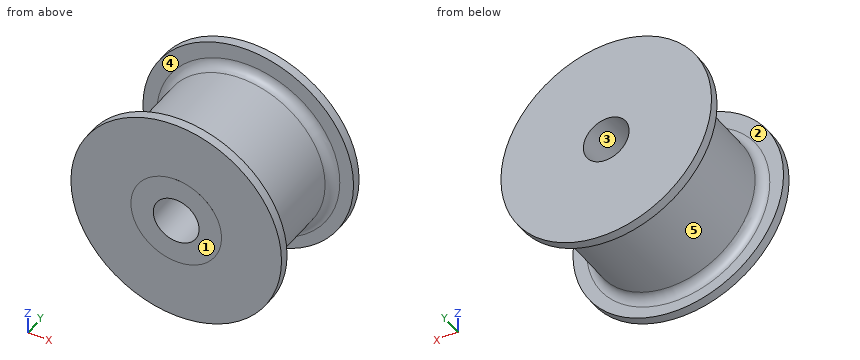
```python
from build123d import *

# Parameters (mm, degrees)
SKETCH1_R           = 4.95
BOSS_EXTRUDE2_DEPTH = 0.001
SKETCH4_R           = 11.5
BOSS_EXTRUDE3_DEPTH = 1
SKETCH5_R           = 9
BOSS_EXTRUDE4_DEPTH = 12
SKETCH6_R           = 11.5
BOSS_EXTRUDE5_DEPTH = 1
FILLET1_R           = 1
FILLET2_R           = 1
SKETCH7_R           = 2.5
CUT_EXTRUDE1_DEPTH  = 15.001


with BuildPart() as part:
    # Sketch1 → Boss-Extrude2 (new body)
    with BuildSketch(Plane(origin=(0, 0, 0), x_dir=(1, 0, 0), z_dir=(0, 1, 0))):
        Circle(SKETCH1_R)
    extrude(amount=BOSS_EXTRUDE2_DEPTH)

    # Sketch4 → Boss-Extrude3 (add)
    with BuildSketch(Plane(origin=(0, 0.001, 0), x_dir=(1, 0, 0), z_dir=(0, 1, 0))):
        Circle(SKETCH4_R)
    extrude(amount=BOSS_EXTRUDE3_DEPTH)

    # Sketch5 → Boss-Extrude4 (add)
    with BuildSketch(Plane(origin=(0, 1.001, 0), x_dir=(1, 0, 0), z_dir=(0, 1, 0))):
        with Locations((0, 0.291114712)):
            Circle(SKETCH5_R)
    extrude(amount=BOSS_EXTRUDE4_DEPTH)

    # Sketch6 → Boss-Extrude5 (add)
    with BuildSketch(Plane(origin=(0, 13.001, 0), x_dir=(1, 0, 0), z_dir=(0, 1, 0))):
        Circle(SKETCH6_R)
    extrude(amount=BOSS_EXTRUDE5_DEPTH)

    # Fillet1
    fillet1_edges = [part.edges().sort_by_distance(p)[0] for p in [
        (-9, 1.001, -0.291114712),
    ]]
    fillet(fillet1_edges, radius=FILLET1_R)

    # Fillet2
    fillet2_edges = [part.edges().sort_by_distance(p)[0] for p in [
        (-9, 13.001, -0.291114712),
    ]]
    fillet(fillet2_edges, radius=FILLET2_R)

    # Sketch7 → Cut-Extrude1 (cut, through all)
    with BuildSketch(Plane.XZ):
        Circle(SKETCH7_R)
    extrude(amount=-CUT_EXTRUDE1_DEPTH, mode=Mode.SUBTRACT)


solid = part.part
```
Here's how the part is built. I have some questions about the finished solid (model axes, mm). Face numbers are marked on the shaded views. A direction names the side the tool comes from. Give positions to 0.01 mm unless a question says otherwise; leave off trailing zeros. Loops run counter-clockwise (first coordinate to the right, second up) from the corner with the lowest first, then second, coordinate; pieces in that order, holes last. Notation, with made-up numbers: (16.5, 65) -> (57.5, 65) arc R6 cw to (57.5, 71) -> close; hole circle Ø7 at (-23.75, 42.25). An arc over 180 degrees is marked (long way). Use one line per item in the form item = value. Start each with the question number.
1) Thinking about a two-plate mould opening in Z: for the marked faces 3, 4 and 5, which applies, +Z half, -Z half, draft (parallel to the pull), parting line (faces both ways), or undercut?
2) For P1, Ø3, axis at x = 7, y = 10.5, coming from the -Z side (3 decimals); P2, Ø5, axis at y = 6.5, z = -4, coming from the -X side; P3, Ø3, axis at y = 9, z = 4.5, coming from the +X side, each with a flat end and sliding along its axis, tell me the tip position at first contact or that it passes through.
3) Imagine slicing it at B-B (y = 3.5). Please give me the cut outline in (x, z), then the cut area to 3 significant figures.
4) Which directions (+Z, -Z, +X, -X, +Y, -Y) give clear straight access to the entire face, cutting with the end or side of a thin tool? Please do the marked faces 1 and 2.
5) Please list where these lines run through material, in increasing order: line 1 along Y through (x, z) = (3, 9.5); line 2 along Z through (x, y) = (0, 8.75); line 3 along X through (y, z) = (8.25, -0.5).
Check values:
q1.face_3 = undercut
q1.face_4 = draft
q1.face_5 = parting line
q2.P1 = -7.415
q2.P2 = -8.92
q2.P3 = 8.38
q3.outline = circle Ø18 at (0, -0.29); hole circle Ø5 at (0, 0)
q3.area = 235 mm^2
q4.face_1 = +Z, -Z, +X, -X, -Y
q4.face_2 = none
q5.line_1 = 0 to 1, 13 to 14
q5.line_2 = -9.29 to -2.5, 2.5 to 8.71
q5.line_3 = -9 to -2.45, 2.45 to 9
